The figure shows three views and two pictorial views of one solid part (mm, origin at its lowest corner). Answer the questions. Give positions to 0.01 mm unless a question says otherwise; leave off trailing zeros. Write each loop counter-clockwise with the first axis right and the second up, starting at its lowest first coordinate (ties: lowest second). Pieces come first, ordered by that corner, then holes. Notation, with made-up numbers: M 48.5,10 L 81.5,10 A23 ccw 81.5,39 Z; hole C 32,7 d4. An arc over 180 degrees is marked long. Return JSON: item names as keys, results as strings.
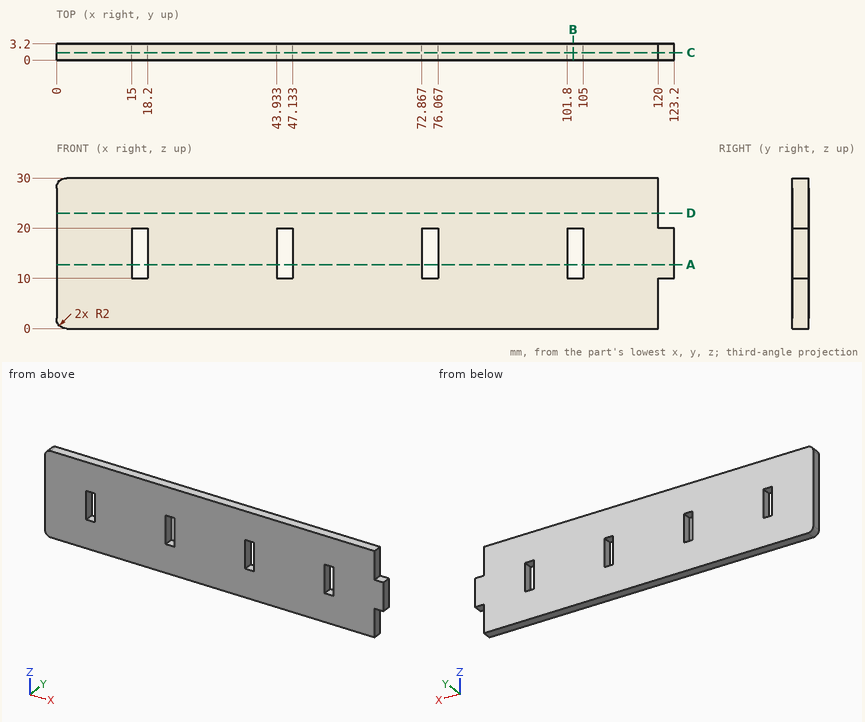
Item 1: A cutting plane is placed at C-C, the plane y = 1.5. Write down the section's boundary in (x, z).
Geometry results:
{"outline": "M 0,2 A2 ccw 2,0 L 120,0 L 120,10 L 123.2,10 L 123.2,20 L 120,20 L 120,30 L 2,30 A2 ccw 0,28 Z; hole M 15,10 L 18.2,10 L 18.2,20 L 15,20 Z; hole M 43.93,10 L 47.13,10 L 47.13,20 L 43.93,20 Z; hole M 72.87,10 L 76.07,10 L 76.07,20 L 72.87,20 Z; hole M 101.8,10 L 105,10 L 105,20 L 101.8,20 Z"}
Item 2: Find the intervals of material crossed by line 1 (X direction, y = 1.05, z = 10.75); line 2 (Z direction, x = 17, y = 2.65); line 3 (X direction, y = 1, z = 3.5), in increasing order.
Geometry results:
{"line 1": "x = 0 to 15, 18.2 to 43.93, 47.13 to 72.87, 76.07 to 101.8, 105 to 123.2", "line 2": "z = 0 to 10, 20 to 30", "line 3": "x = 0 to 120"}
Item 3: Given pin 1 Ø1.6 at (x, y) = (102.5, 2.5) entering from -Z; pin 2 Ø1 at (x, y) = (121, 1) entering from +Z; pin 3 Ø1.6 at (y, z) = (1, 6.5) entering from +X, each flat-ended and moving along its own axis, determine where each tip first touches the part or whether it passes through.
Geometry results:
{"pin 1": "stops at z = 0", "pin 2": "stops at z = 20", "pin 3": "stops at x = 120"}
Item 4: A cutting plane is placed at D-D, the plane z = 23. Write down the section's boundary in (x, y).
Geometry results:
{"outline": "M 0,0 L 120,0 L 120,3.2 L 0,3.2 Z"}
Item 5: A cutting plane is placed at A-A, the plane z = 12.75. Write down the section's boundary in (x, y).
Geometry results:
{"outline": "M 0,0 L 15,0 L 15,3.2 L 0,3.2 Z; M 18.2,0 L 43.93,0 L 43.93,3.2 L 18.2,3.2 Z; M 47.13,0 L 72.87,0 L 72.87,3.2 L 47.13,3.2 Z; M 76.07,0 L 101.8,0 L 101.8,3.2 L 76.07,3.2 Z; M 105,0 L 123.2,0 L 123.2,3.2 L 105,3.2 Z"}
Item 6: A cutting plane is placed at B-B, the plane x = 103. Write down the section's boundary in (y, z), plus the area to 3 significant figures.
Geometry results:
{"outline": "M 0,0 L 3.2,0 L 3.2,10 L 0,10 Z; M 0,20 L 3.2,20 L 3.2,30 L 0,30 Z", "area": "64.0 mm2"}
